```python
from build123d import *

# Parameters (mm, degrees)
SKETCH1_W           = 34
SKETCH1_H           = 64
BOSS_EXTRUDE1_DEPTH = 9.04
SKETCH2_W           = 5
SKETCH2_H           = 21
BOSS_EXTRUDE2_DEPTH = 25
SKETCH3_R           = 1.6
SKETCH3_R_2         = 3
CUT_EXTRUDE1_DEPTH  = 30
SKETCH4_R           = 1.6
CUT_EXTRUDE2_DEPTH  = 10
SKETCH5_R           = 3.5
CUT_EXTRUDE3_DEPTH  = 10


with BuildPart() as part:
    # Sketch1 → Boss-Extrude1 (new body)
    with BuildSketch(Plane.XY):
        Rectangle(SKETCH1_W, SKETCH1_H)
    extrude(amount=BOSS_EXTRUDE1_DEPTH)

    # Sketch2 → Boss-Extrude2 (add)
    with BuildSketch(Plane.XY.offset(9.04)):
        with Locations((12, 3.7)):
            Rectangle(SKETCH2_W, SKETCH2_H)
        with Locations((-12, 3.7)):
            Rectangle(SKETCH2_W, SKETCH2_H)
    extrude(amount=BOSS_EXTRUDE2_DEPTH)

    # Sketch3 → Cut-Extrude1 (cut)
    with BuildSketch(Plane(origin=(14.5, 0, 0), x_dir=(0, 0, -1), z_dir=(1, 0, 0))):
        with Locations((-28.54, 0.2)):
            Circle(SKETCH3_R)
        with Locations((-11.04, 0.2)):
            Circle(SKETCH3_R)
        with Locations((-19.79, 9.8)):
            Circle(SKETCH3_R_2)
    extrude(amount=-CUT_EXTRUDE1_DEPTH, mode=Mode.SUBTRACT)

    # Sketch4 → Cut-Extrude2 (cut)
    with BuildSketch(Plane.XY.offset(9.04)):
        with Locations((-14, -27)):
            Circle(SKETCH4_R)
        with Locations((-14, 27)):
            Circle(SKETCH4_R)
        with Locations((14, -27)):
            Circle(SKETCH4_R)
        with Locations((14, 27)):
            Circle(SKETCH4_R)
    extrude(amount=-CUT_EXTRUDE2_DEPTH, mode=Mode.SUBTRACT)

    # Sketch5 → Cut-Extrude3 (cut)
    with BuildSketch(Plane(origin=(0, 0, 0), x_dir=(-1, 0, 0), z_dir=(0, 0, -1))):
        with Locations((-0.5, 26.8)):
            Circle(SKETCH5_R)
        with Locations((-10.5, 26.8)):
            Circle(SKETCH5_R)
        with Locations((-0.5, -11.2)):
            Circle(SKETCH5_R)
        with Locations((-10.5, -11.2)):
            Circle(SKETCH5_R)
    extrude(amount=-CUT_EXTRUDE3_DEPTH, mode=Mode.SUBTRACT)


solid = part.part
```
Source: CAD feature listing. Evaluate the final solid. Frame: model axes, mm. A direction names the side the tool comes from. Round coordinates to 2 decimals unless told otherwise and drop trailing zeros. Loops run counter-clockwise (first coordinate to the right, second up) from the corner with the lowest first, then second, coordinate; pieces in that order, holes last.
1. Section query B-B on x = 10.5. Output: boundary loops of the cut face in (y, z).
2. Ray query, L1, parallel to Y at x = 10.5, z = 5.5; L2, parallel to Y at x = -14, z = 3; L3, parallel to X at y = 11, z = 12.5. Return the intervals inside material, ascending.
3. Section query C-C on y = 0.2. Output: boundary loops of the cut face in (x, z), and give its area (3 significant figures).
4. Access query for faces 5 (the flat face through (-12, 14.2, 21)), 6 (the flat face through (-12, 4, 34.04)), 7 (the flat face through (9.5, 4, 21)). Directions: +Z, -Z, +X, -X, +Y, -Y. A direction counts if a zero-diameter tool reaches every point of the face in a straight line with its end or side. Return the directions, or none.
5. Section query A-A on z = 19.79. Output: boundary loops of the cut face in (x, y), and give its area (3 significant figures).
6. Section query D-D on z = 24. Output: boundary loops of the cut face in (x, y).
7. Mould query, pull axis Y, two halves, no side actions, for faces 1 (the flat face through (14.5, 4, 21)), 2 (the cylindrical face through (-1.115, 23.695, 4.457)), 3 (the flat face through (12, -6.8, 21)), 4 (the flat face through (0, 32, 4)). Classes: released by +Y, released by -Y, zero draft, split by the parting line, or undercut.
8. Contact query for flat-ended pins moving along their axis: pin 1 (4 mm diameter, centred on x = -13, z = 23.5, fed in from -Y); pin 2 (8 mm diameter, centred on y = 1, z = 22, fed in from -X); pin 3 (3 mm diameter, centred on x = -0.5, y = -15.5, fed in from +Z). Output: stop coordinate, or through.
Answers below:
1. outline: (-32, 0) - (-14.7, 0) - (-14.7, 9.04) - (-32, 9.04) - close; (-7.7, 0) - (23.3, 0) - (23.3, 9.04) - (14.2, 9.04) - (14.2, 34.04) - (-6.8, 34.04) - (-6.8, 9.04) - (-7.7, 9.04) - close; (30.3, 0) - (32, 0) - (32, 9.04) - (30.3, 9.04) - close; hole circle Ø3.2 at (0.2, 11.04); hole circle Ø3.2 at (0.2, 28.54); hole circle Ø6 at (9.8, 19.79)
2. L1: y = -32 to -14.7, -7.7 to 23.3, 30.3 to 32
2. L2: y = -32 to -28.6, -25.4 to 25.4, 28.6 to 32
2. L3: x = -14.5 to -9.5, 9.5 to 14.5
3. outline: (-17, 0) - (17, 0) - (17, 9.04) - (14.5, 9.04) - (14.5, 9.44) - (9.5, 9.44) - (9.5, 9.04) - (-9.5, 9.04) - (-9.5, 9.44) - (-14.5, 9.44) - (-14.5, 9.04) - (-17, 9.04) - close; (-14.5, 12.64) - (-9.5, 12.64) - (-9.5, 26.94) - (-14.5, 26.94) - close; (-14.5, 30.14) - (-9.5, 30.14) - (-9.5, 34.04) - (-14.5, 34.04) - close; (9.5, 12.64) - (14.5, 12.64) - (14.5, 26.94) - (9.5, 26.94) - close; (9.5, 30.14) - (14.5, 30.14) - (14.5, 34.04) - (9.5, 34.04) - close
3. area: 493 mm2
4. face 5: +Z, +X, -X, +Y
4. face 6: +Z, +X, -X, +Y, -Y
4. face 7: +Z, +Y, -Y
5. outline: (-14.5, -6.8) - (-9.5, -6.8) - (-9.5, 6.8) - (-14.5, 6.8) - close; (-14.5, 12.8) - (-9.5, 12.8) - (-9.5, 14.2) - (-14.5, 14.2) - close; (9.5, -6.8) - (14.5, -6.8) - (14.5, 6.8) - (9.5, 6.8) - close; (9.5, 12.8) - (14.5, 12.8) - (14.5, 14.2) - (9.5, 14.2) - close
5. area: 150 mm2
6. outline: (-14.5, -6.8) - (-9.5, -6.8) - (-9.5, 14.2) - (-14.5, 14.2) - close; (9.5, -6.8) - (14.5, -6.8) - (14.5, 14.2) - (9.5, 14.2) - close
7. face 1: zero draft
7. face 2: undercut
7. face 3: released by -Y
7. face 4: released by +Y
8. pin 1: stops at y = -6.8
8. pin 2: stops at x = -14.5
8. pin 3: stops at z = 9.04
